For this review, take the finished solid that the model builds, in its own axes (mm). A direction names the side the tool comes from. Round coordinates to 2 decimals unless told otherwise and drop trailing zeros. Order: outer loops, then holes, each group sorted by start corner. A loop starts at its lowest first (then second) coordinate and runs counter-clockwise, first axis right, second up. Notation, with made-up numbers: (86.25, 68.5) -> (103.25, 68.5) arc R25 ccw to (103.25, 83.5) -> close; hole circle Ø9 at (-14, 34.5). An arc over 180 degrees is marked (long way). Answer in a Markdown table with one row per item.
```python
from build123d import *

# Parameters (mm, degrees)
F1_DEPTH = 12.7
F3_DEPTH = 21.59


with BuildPart() as f1:
    # F0 (on Top) → F1 (new body)
    with BuildSketch(Plane.XY):
        Polygon((33.208514, -8.155814), (33.208514, 21.379727), (-30.508613, 21.379727), (-42.787436, 17.397408), (-42.787436, -4.173495), (-30.508613, -8.155814), align=None)
        Polygon((33.208514, -8.155814), (50.465232, 6.611957), (33.208514, 21.379727), align=None)
        Polygon((49.4617, 6.611957), (41.17628, 0), (34.235716, -5.939522), (34.235716, 6.611957), (34.235716, 19.163436), (41.17628, 13.223914), align=None, mode=Mode.SUBTRACT)
    extrude(amount=F1_DEPTH)

    # F2 (on face) → F3 (cut)
    with BuildSketch(Plane(origin=(-42.787436, 0, 0), x_dir=(0, -1, 0), z_dir=(-1, 0, 0))):
        Polygon((-15.368456, 11.105623), (-15.368456, 6.35), (-15.368456, 1.594377), (2.144542, 1.594377), (2.144542, 6.35), (2.144542, 11.105623), align=None)
    extrude(amount=-F3_DEPTH, mode=Mode.SUBTRACT)


solid = f1.part
```
Q1. Take a section at D-D, the plane x = 44. Write out the cut boundary in (y, z), then the cut area to 3 significant figures.
Answer key:
| item | result |
|---|---|
| outline | (1.08, 0) -> (2.25, 0) -> (2.25, 12.7) -> (1.08, 12.7) -> close; (10.97, 0) -> (12.14, 0) -> (12.14, 12.7) -> (10.97, 12.7) -> close |
| area | 29.8 mm^2 |
Q2. The part is to be moulded in two halves that separate along Z. For faces 4 (the face through (-21.197, 7, 6)), 5 (the face through (45.377, 3.352, 6.261)), 6 (the face through (-7, 7, 12.7)), 7 (the face through (-32, 15.368, 6)), say which applies: +Z half, -Z half, draft (parallel to the pull), parting line (faces both ways), or undercut.
Answer key:
| item | result |
|---|---|
| face 4 | undercut |
| face 5 | draft |
| face 6 | +Z half |
| face 7 | undercut |
Q3. Take a section at C-C, the plane z = 6.25. Write out the cut boundary in (x, y), then the cut area to 3 significant figures.
Answer key:
| item | result |
|---|---|
| outline | (-42.79, -4.17) -> (-30.51, -8.16) -> (33.21, -8.16) -> (50.47, 6.61) -> (33.21, 21.38) -> (-30.51, 21.38) -> (-42.79, 17.4) -> (-42.79, 15.37) -> (-21.2, 15.37) -> (-21.2, -2.14) -> (-42.79, -2.14) -> close; hole (34.24, -5.94) -> (41.18, 0) -> (49.46, 6.61) -> (41.18, 13.22) -> (34.24, 19.16) -> close |
| area | 1,880 mm^2 |
Q4. Take a section at B-B, the plane y = 12.25. Write out the cut boundary in (x, z), then the cut area to 3 significant figures.
Answer key:
| item | result |
|---|---|
| outline | (-42.79, 0) -> (34.24, 0) -> (34.24, 12.7) -> (-42.79, 12.7) -> (-42.79, 11.11) -> (-21.2, 11.11) -> (-21.2, 1.59) -> (-42.79, 1.59) -> close; (42.4, 0) -> (43.88, 0) -> (43.88, 12.7) -> (42.4, 12.7) -> close |
| area | 792 mm^2 |
Q5. Tool access review of faces 1 (the face through (-36.562, 19.416, 6.261)), 2 (the face through (34.236, 6, 6)), 3 (the face through (-32, 6, 11.106)): name each direction out of +Z, -Z, +X, -X, +Y, -Y from which nothing blocks a thin tool from reaching the whole face with its end or side.
Answer key:
| item | result |
|---|---|
| face 1 | +Z, -Z, -X, +Y |
| face 2 | +Z, -Z |
| face 3 | -X |
Q6. Take a section at A-A, the plane x = -28. Write out the cut boundary in (y, z), then the cut area to 3 significant figures.
Answer key:
| item | result |
|---|---|
| outline | (-8.16, 0) -> (21.38, 0) -> (21.38, 12.7) -> (-8.16, 12.7) -> close; hole (-2.14, 1.59) -> (15.37, 1.59) -> (15.37, 11.11) -> (-2.14, 11.11) -> close |
| area | 209 mm^2 |
Q7. To check wall thickness, follow probe 1 along Y at (x, z) = (-30, 7.75); probe 2 along Z at (x, y) = (-33, 1.5); probe 3 along Y at (x, z) = (43, 3.5). State the ranges of each line that lie inside material, in increasing order.
Answer key:
| item | result |
|---|---|
| probe 1 | y = -8.16 to -2.14, 15.37 to 21.38 |
| probe 2 | z = 0 to 1.59, 11.11 to 12.7 |
| probe 3 | y = 0.22 to 1.46, 11.77 to 13 |
Q8. Clearance check with flat-ended pins moving along their axes: pin 1 Ø3 at (x, z) = (41, 4) entering from +Y; pin 2 Ø2 at (y, z) = (6.5, 4.5) entering from -X; pin 3 Ø5 at (x, z) = (-36, 8) entering from +Y; pin 4 Ø1.5 at (x, y) = (-14, 11) entering from -Z. State where each tip first meets the part, or that it passes through.
Answer key:
| item | result |
|---|---|
| pin 1 | stops at y = 16 |
| pin 2 | stops at x = -21.2 |
| pin 3 | stops at y = 20.41 |
| pin 4 | stops at z = 0 |
